Study the drawing (mm; zero at the part's minimum x, y, z) and answer. A direction names the side the tool comes from. Coordinates: 2 decimals unless noted, no trailing zeros. Write each loop counter-clockwise with the first axis right and the second up, starting at its lowest first coordinate (ties: lowest second). Pieces come first, ordered by that corner, then holes. Notation, with made-up numbers: M 15,28.25 L 51,28.25 A27 ccw 51,54.25 Z; hole C 79.25,30.5 d7. An arc over 180 degrees is marked long. Answer as CSV lines item,"result". Start each with the question number.
(1) A cutting plane is placed at D-D on y = 37. Give the vertices of the cut face in (x, z) (1 decimal).
(2) Find the intervals of material crossed by L1, parallel to Z at x = 16, y = 26 (1 decimal); L2, parallel to Y at x = 12.7, z = 1.05 (1 decimal), in increasing order. Write a range as [from, to].
(3) A cutting plane is placed at C-C on y = 46. Give the vertices of the cut face in (x, z) (1 decimal).
(4) For the marked faces 4 and 5, determine the directions among +Z, -Z, +X, -X, +Y, -Y from which every point of the face is accessible in a straight line to the end or side of a thin tool.
(5) The mould has two halves that part along X. Classify the marked faces 1, 2 and 3: released by +X, released by -X, zero draft, split by the parting line, or undercut.
(6) Flat-ended cylindrical pins translate along their axes: P1, Ø12.5, axis at x = 14, z = 22, coming from the +Y side (1 decimal); P2, Ø1, axis at x = 8.5, y = 54.5, coming from the -Z side; P3, Ø7.5, axis at x = 13, y = 30.5, coming from the +Z side (1 decimal). Find the tip coordinate at first contact, or state that the pin passes through.
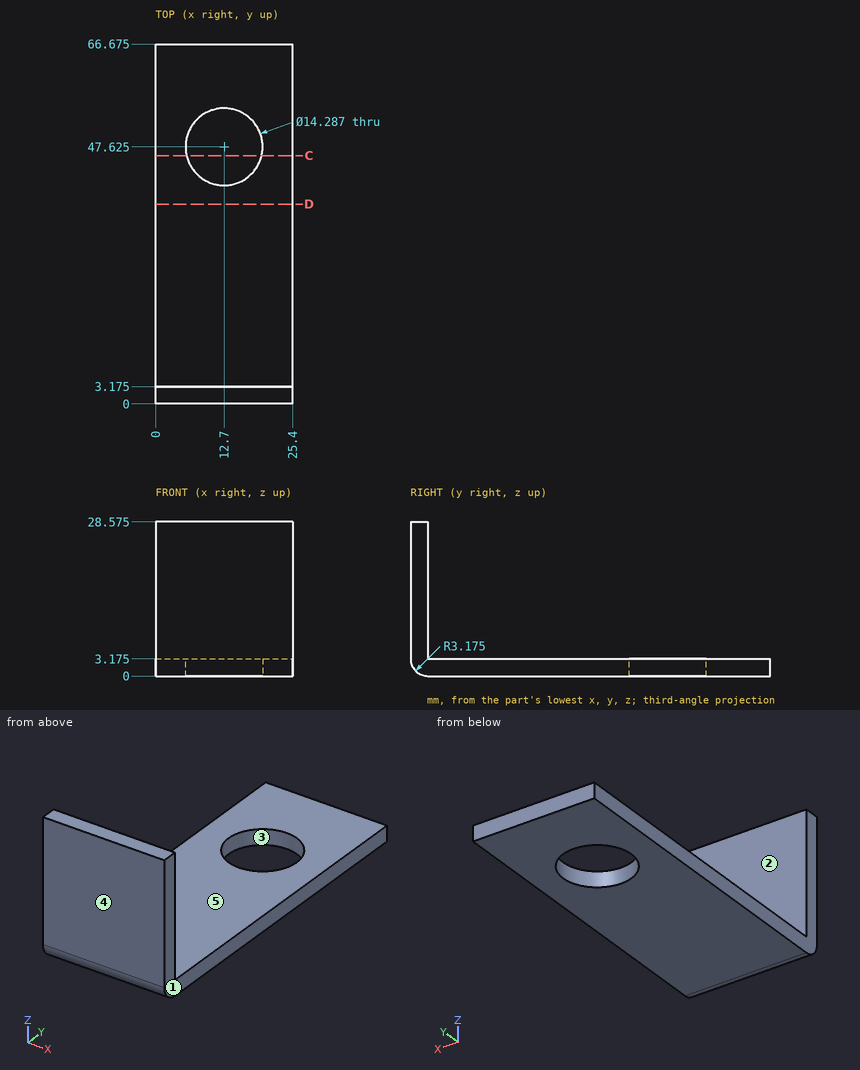
Here are the results:
1,outline,"M 0,0 L 25.4,0 L 25.4,3.2 L 0,3.2 Z"
2,L1,"z = [0, 3.2]"
2,L2,"y = [0.8, 40.5], [54.8, 66.7]"
3,outline,"M 0,0 L 5.7,0 L 5.7,3.2 L 0,3.2 Z; M 19.7,0 L 25.4,0 L 25.4,3.2 L 19.7,3.2 Z"
4,face 4,"+Z, -Z, +X, -X, -Y"
4,face 5,"+Z, +X, -X, +Y"
5,face 1,"released by +X"
5,face 2,"zero draft"
5,face 3,"undercut"
6,P1,"stops at y = 3.2"
6,P2,"stops at z = 0"
6,P3,"stops at z = 3.2"
